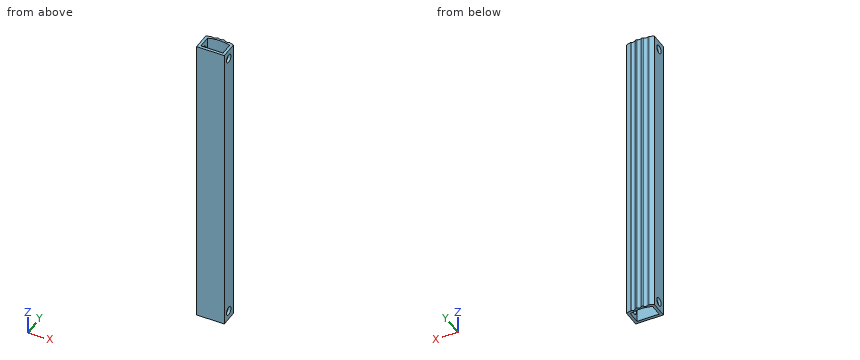
```python
from build123d import *

# Parameters (mm, degrees)
BOSS_EXTRU_1_DEPTH      = 54.5
ESQUISSE2_R             = 1.5
ENL_V_MAT_EXTRU_1_DEPTH = 56.87007968


with BuildPart() as part:
    # Esquisse1 → Boss.-Extru.1 (new, symmetric)
    with BuildSketch(Plane.XY):
        with BuildLine():
            Line((-5, 0), (5, 0))
            Line((5, 0), (5, 6.2))
            ThreePointArc((5, 6.2), (4.198380709, 6.503397881), (3.378511037, 6.753312837))
            ThreePointArc((3.378511037, 6.753312837), (3.182940128, 6.766167342), (2.997453176, 6.702860077))
            ThreePointArc((2.997453176, 6.702860077), (2.185788495, 6.558879309), (1.472744558, 6.972519685))
            ThreePointArc((1.472744558, 6.972519685), (1.320223309, 7.095607002), (1.132107007, 7.150611326))
            ThreePointArc((1.132107007, 7.150611326), (1.107721314, 7.152719926), (1.083331695, 7.154782609))
            ThreePointArc((1.083331695, 7.154782609), (0.899623928, 7.135921685), (0.735293006, 7.051662404))
            ThreePointArc((0.735293006, 7.051662404), (0, 6.8), (-0.735293006, 7.051662404))
            ThreePointArc((-0.735293006, 7.051662404), (-0.899623928, 7.135921685), (-1.083331695, 7.154782609))
            ThreePointArc((-1.083331695, 7.154782609), (-1.107721314, 7.152719926), (-1.132107007, 7.150611326))
            ThreePointArc((-1.132107007, 7.150611326), (-1.320223309, 7.095607002), (-1.472744558, 6.972519685))
            ThreePointArc((-1.472744558, 6.972519685), (-2.185788495, 6.558879309), (-2.997453176, 6.702860077))
            ThreePointArc((-2.997453176, 6.702860077), (-3.182940128, 6.766167342), (-3.378511037, 6.753312837))
            ThreePointArc((-3.378511037, 6.753312837), (-4.198380709, 6.503397881), (-5, 6.2))
            Line((-5, 6.2), (-5, 0))
        make_face()
        with BuildLine():
            Line((-4, 1), (-4, 5.513708499))
            ThreePointArc((-4, 5.513708499), (0, 6.2), (4, 5.513708499))
            Line((4, 5.513708499), (4, 1))
            Line((4, 1), (-4, 1))
        make_face(mode=Mode.SUBTRACT)
    extrude(amount=BOSS_EXTRU_1_DEPTH, both=True)

    # Esquisse2 → Enlèv. mat.-Extru.1 (cut, through all)
    with BuildSketch(Plane.ZY.offset(5)):
        with Locations((-51.25, 3)):
            Circle(ESQUISSE2_R)
        with Locations((51.25, 3)):
            Circle(ESQUISSE2_R)
    extrude(amount=-ENL_V_MAT_EXTRU_1_DEPTH, mode=Mode.SUBTRACT)


solid = part.part
```
Part model, mm, in its own coordinate system. Round coordinates to 2 decimals unless told otherwise and drop trailing zeros. Write each loop counter-clockwise with the first axis right and the second up, starting at its lowest first coordinate (ties: lowest second). Pieces come first, ordered by that corner, then holes.
Item 1: Cut at A-A, the plane y = 3. Give the cut face in (x, z).
Results:
outline: (-5, -54.5) - (-4, -54.5) - (-4, -52.75) - (-5, -52.75) - close; (-5, -49.75) - (-4, -49.75) - (-4, 49.75) - (-5, 49.75) - close; (-5, 52.75) - (-4, 52.75) - (-4, 54.5) - (-5, 54.5) - close; (4, -54.5) - (5, -54.5) - (5, -52.75) - (4, -52.75) - close; (4, -49.75) - (5, -49.75) - (5, 49.75) - (4, 49.75) - close; (4, 52.75) - (5, 52.75) - (5, 54.5) - (4, 54.5) - close
Item 2: Cut at C-C, the plane z = -38. Give the cut face in (x, y).
Results:
outline: (-5, 0) - (5, 0) - (5, 6.2) arc R13 ccw to (3.38, 6.75) arc R0.5 ccw to (3, 6.7) arc R1.2 cw to (1.47, 6.97) arc R0.5 ccw to (1.13, 7.15) arc R13 ccw to (1.08, 7.15) arc R0.5 ccw to (0.74, 7.05) arc R1.2 cw to (-0.74, 7.05) arc R0.5 ccw to (-1.08, 7.15) arc R13 ccw to (-1.13, 7.15) arc R0.5 ccw to (-1.47, 6.97) arc R1.2 cw to (-3, 6.7) arc R0.5 ccw to (-3.38, 6.75) arc R13 ccw to (-5, 6.2) - close; hole (-4, 1) - (4, 1) - (4, 5.51) arc R12 ccw to (-4, 5.51) - close
Item 3: Cut at B-B, the plane z = -51.25. Give the cut face in (x, y).
Results:
outline: (-5, 0) - (5, 0) - (5, 1.5) - (4, 1.5) - (4, 1) - (-4, 1) - (-4, 1.5) - (-5, 1.5) - close; (-5, 4.5) - (-4, 4.5) - (-4, 5.51) arc R12 cw to (4, 5.51) - (4, 4.5) - (5, 4.5) - (5, 6.2) arc R13 ccw to (3.38, 6.75) arc R0.5 ccw to (3, 6.7) arc R1.2 cw to (1.47, 6.97) arc R0.5 ccw to (1.13, 7.15) arc R13 ccw to (1.08, 7.15) arc R0.5 ccw to (0.74, 7.05) arc R1.2 cw to (-0.74, 7.05) arc R0.5 ccw to (-1.08, 7.15) arc R13 ccw to (-1.13, 7.15) arc R0.5 ccw to (-1.47, 6.97) arc R1.2 cw to (-3, 6.7) arc R0.5 ccw to (-3.38, 6.75) arc R13 ccw to (-5, 6.2) - close
Item 4: Probe L1, parallel to X at y = 2.5, z = -1; L2, parallel to Y at x = -4.15, z = 51.25; L3, parallel to Y at x = -3, z = -48.5. List the from-to ranges inside material, lowest first.
Results:
L1: x = -5 to -4, 4 to 5
L2: y = 0 to 1.5, 4.5 to 6.52
L3: y = 0 to 1, 5.82 to 6.7
